```python
from build123d import *

# Parameters (mm, degrees)
F0_W        = 68.9248368144
F0_H        = 38.2718367036
F1_DEPTH    = 92.964
F2_R        = 4.2924717139
F3_R        = 5.08
F4_T1_DEPTH = 108.9915282861
F6_DEPTH    = 66.294
F7_R        = 5.08


# Not quite as in the source:
# - a fillet or chamfer that OpenCascade refuses, or shapes differently, is made with other operations: its cross-section is extruded or revolved along the edge and cut away or added


with BuildPart() as f1:
    # F0 (on Top) → F1 (new body)
    with BuildSketch(Plane.XY):
        Polygon((-76.8856033683, 47.9822456837), (-76.8856033683, -11.9746578857), (64.6745637059, -11.9746578857), (64.6745637059, -2.9509027954), (64.6745637059, 35.3209339082), (64.6745637059, 47.9822456837), align=None)
        with Locations((99.1369821131, 16.1850155564)):
            Rectangle(F0_W, F0_H)
    extrude(amount=F1_DEPTH)

    # F2
    f2_edges = [f1.edges().sort_by_distance(p)[0] for p in [
        (-76.885603, 18.003794, 92.964),
        (-6.10552, -11.974658, 92.964),
        (64.674564, -7.46278, 92.964),
        (99.136982, -2.950903, 92.964),
        (133.599401, 16.185016, 92.964),
        (99.136982, 35.320934, 92.964),
        (64.674564, 41.65159, 92.964),
        (-6.10552, 47.982246, 92.964),
    ]]
    fillet(f2_edges, radius=F2_R)

    # F3
    f3_edges = [f1.edges().sort_by_distance(p)[0] for p in [
        (99.136982, -2.950903, 0),
        (-76.885603, 18.003794, 0),
        (-6.10552, -11.974658, 0),
        (64.674564, -7.46278, 0),
        (133.599401, 16.185016, 0),
        (99.136982, 35.320934, 0),
        (64.674564, 41.65159, 0),
        (-6.10552, 47.982246, 0),
    ]]
    fillet(f3_edges, radius=F3_R)

    # F4: fillet of radius 5.08 on 4 edges, made by hand

    # F4_s2 → F4_t1 (cut)
    with BuildSketch(Plane.XY.offset(-7.62)):
        with BuildLine():
            ThreePointArc((-76.8856033683, 42.9022456837), (-75.3977058167, 46.4943481321), (-71.8056033683, 47.9822456837))
            Line((-71.8056033683, 47.9822456837), (-76.8856033683, 47.9822456837))
            Line((-76.8856033683, 47.9822456837), (-76.8856033683, 42.9022456837))
        make_face()
        with BuildLine():
            ThreePointArc((-76.8856033683, -6.8946578857), (-75.3977058167, -10.4867603342), (-71.8056033683, -11.9746578857))
            Line((-71.8056033683, -11.9746578857), (-76.8856033683, -11.9746578857))
            Line((-76.8856033683, -11.9746578857), (-76.8856033683, -6.8946578857))
        make_face()
    extrude(amount=F4_T1_DEPTH, mode=Mode.SUBTRACT)

    # F5 (on face) → F6 (cut)
    with BuildSketch(Plane(origin=(0, 47.9822456837, 0), x_dir=(-1, 0, 0), z_dir=(0, 1, 0))):
        Polygon((34.4493128359, 24.1737514734), (34.9953584373, 71.4389234781), (-5.412035156, 71.4389234781), (-32.1682840586, 48.3612157404), (-5.412035156, 24.1737514734), align=None)
    extrude(amount=-F6_DEPTH, mode=Mode.SUBTRACT)

    # F7
    f7_edges = [f1.edges().sort_by_distance(p)[0] for p in [
        (-34.722336, 47.982246, 47.806337),
        (-34.995358, 18.003794, 71.438923),
        (-34.722336, -11.974658, 47.806337),
        (-34.449313, 18.003794, 24.173751),
        (18.79016, 47.982246, 59.90007),
        (32.168284, 18.003794, 48.361216),
        (18.79016, -11.974658, 59.90007),
        (5.412035, 18.003794, 71.438923),
        (18.79016, 47.982246, 36.267484),
        (5.412035, 18.003794, 24.173751),
        (18.79016, -11.974658, 36.267484),
        (-14.791662, -11.974658, 71.438923),
        (-14.518639, -11.974658, 24.173751),
        (-14.518639, 47.982246, 24.173751),
        (-14.791662, 47.982246, 71.438923),
    ]]
    fillet(f7_edges, radius=F7_R)


solid = f1.part
```
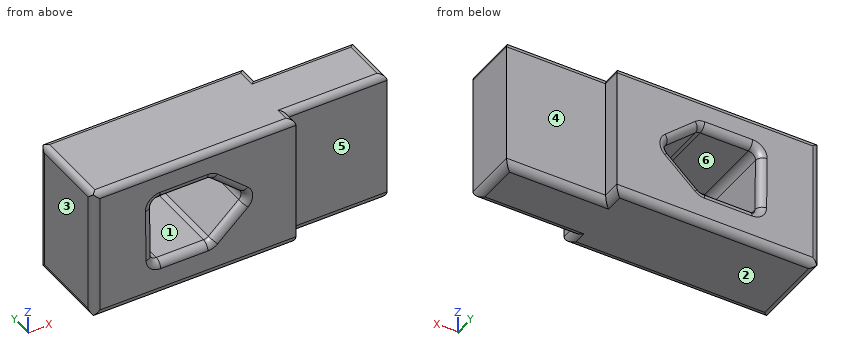
Work out the finished part from the listing and answer in its coordinate system (mm). Face numbers are marked on the shaded views. A direction names the side the tool comes from. Give positions to 0.01 mm unless a question says otherwise; leave off trailing zeros. Order: outer loops, then holes, each group sorted by start corner. A loop starts at its lowest first (then second) coordinate and runs counter-clockwise, first axis right, second up. Notation, with made-up numbers: (62.25, 54.5) -> (114.25, 54.5) arc R35 cw to (114.25, 93.5) -> close; hole circle Ø3 at (53, 1). An arc over 180 degrees is marked (long way). Answer as CSV lines item,"result". Start each with the question number.
(1) Which of the six approach directions +Z, -Z, +X, -X, +Y, -Y give full straight-line access (tool end or side, diameter ignored) to the marked faces 4, 5 and 6?
(2) Each of these flat-tipped pins is pushed along its axis until it touches: pin 1 Ø4 at (x, y) = (89.5, -4) entering from -Z; pin 2 Ø6 at (x, z) = (65, 66) entering from -Y; pin 3 Ø6.5 at (y, z) = (43, 54.5) entering from +X; pin 4 Ø5 at (x, z) = (112.5, 68) entering from +Y. Where does it stop, or does it pass through?
(3) For a pull along Z with two mould halves and no side action, classify the marked faces 1, 2 and 3 as released by +Z, released by -Z, zero draft, split by the parting line, or undercut.
(4) Section A-A, the plane x = -15 is taken. Write down the section's boundary in (y, z), plus the area to 3 significant figures.
(5) Section C-C, the plane z = 80.5 is taken. Write down the section's boundary in (x, y).
(6) Section D-D, the plane x = 119.5 is taken. Write down the section's boundary in (y, z).
(7) Section B-B, the plane y = 24 is taken. Write down the section's boundary in (x, z), plus the area to 3 significant figures.
(8) Consider line 1 along Y through (x, z) = (124, 26); line 2 along Z through (x, y) = (-1, 40); line 3 along X through (y, z) = (23.5, 44). Determine where each line is inside the solid, lowest interval first.
Entries:
1,face 4,"+Z, -Z, +X, +Y"
1,face 5,"+Z, -Z, +X, -Y"
1,face 6,"+Y, -Y"
2,pin 1,"z = 2.12"
2,pin 2,"y = -11.97"
2,pin 3,"x = 64.67"
2,pin 4,"y = 35.32"
3,face 1,"undercut"
3,face 2,"released by -Z"
3,face 3,"zero draft"
4,outline,"(-11.97, 5.08) arc R5.08 ccw to (-6.89, 0) -> (42.9, 0) arc R5.08 ccw to (47.98, 5.08) -> (47.98, 19.09) arc R5.08 ccw to (42.9, 24.17) -> (-6.89, 24.17) arc R5.08 ccw to (-11.97, 19.09) -> close; (-11.97, 76.52) arc R5.08 ccw to (-6.89, 71.44) -> (42.9, 71.44) arc R5.08 ccw to (47.98, 76.52) -> (47.98, 88.67) arc R4.29 ccw to (43.69, 92.96) -> (-7.68, 92.96) arc R4.29 ccw to (-11.97, 88.67) -> close"
4,area,"2,700 mm²"
5,outline,"(-76.89, -6.89) arc R5.08 ccw to (-71.81, -11.97) -> (64.67, -11.97) -> (64.67, -2.95) -> (133.6, -2.95) -> (133.6, 35.32) -> (64.67, 35.32) -> (64.67, 47.98) -> (-71.81, 47.98) arc R5.08 ccw to (-76.89, 42.9) -> close"
6,outline,"(-2.95, 5.08) arc R5.08 ccw to (2.13, 0) -> (30.24, 0) arc R5.08 ccw to (35.32, 5.08) -> (35.32, 88.67) arc R4.29 ccw to (31.03, 92.96) -> (1.34, 92.96) arc R4.29 ccw to (-2.95, 88.67) -> close"
7,outline,"(-76.89, 5.08) arc R5.08 ccw to (-71.81, 0) -> (128.52, 0) arc R5.08 ccw to (133.6, 5.08) -> (133.6, 88.67) arc R4.29 ccw to (129.31, 92.96) -> (-72.59, 92.96) arc R4.29 ccw to (-76.89, 88.67) -> close; hole (-34.94, 66.3) -> (-34.51, 29.2) arc R5.08 ccw to (-29.43, 24.17) -> (3.46, 24.17) arc R5.08 ccw to (6.86, 25.49) -> (27.9, 44.5) arc R5.08 ccw to (27.81, 52.12) -> (6.84, 70.21) arc R5.08 ccw to (3.52, 71.44) -> (-29.86, 71.44) arc R5.08 ccw to start"
7,area,"17,000 mm²"
8,line 1,"-2.95 to 35.32"
8,line 2,"0 to 24.17, 71.44 to 92.96"
8,line 3,"-76.89 to -34.68, 27.34 to 133.6"
